Could you check a few things on this drawing? It's one solid part, dimensions in mm from its lowest x, y, z. Round coordinates to 2 decimals unless told otherwise and drop trailing zeros. Order: outer loops, then holes, each group sorted by start corner. A loop starts at its lowest first (then second) coordinate and runs counter-clockwise, first axis right, second up. Notation, with made-up numbers: (-19, 80) -> (6, 80) arc R12 cw to (6, 86) -> close; hole circle Ø1 at (33.5, 86.25). An arc over 180 degrees is marked (long way). Use a Markdown table: item, result. Add a question column.
(1) I want a section at B-B, the plane x = 2.25. Give the number of separate pieces and of enclosed holes in the cut face, then the cut area to 3 significant figures.
(2) If I drill on probe 1 along Y at (x, z) = (5, 6.5); probe 2 along Y at (x, z) = (2.75, 5); probe 3 along Z at (x, y) = (6, 15), over which ranges is the centre line in solid material (lowest first)?
(3) Thinking about a two-plate mould opening in Z: for the marked faces 1, 2, 3 and 4, which applies, pulls with the +Z half, pulls with the -Z half, needs draft (parallel to the pull), parting line crosses it, or undercut?
(4) I want a section at A-A, the plane y = 5.08. Please give me the cut outline in (x, z).
(5) I want a section at C-C, the plane y = 12.75. Please give me the cut outline in (x, z), then the cut area to 3 significant figures.
(6) I'm going to push a flat-ended pin straight in: P1, Ø3, axis at y = 5.08, z = 5.969, coming from the +X side. Where does the tip first touch, or does it pass through?
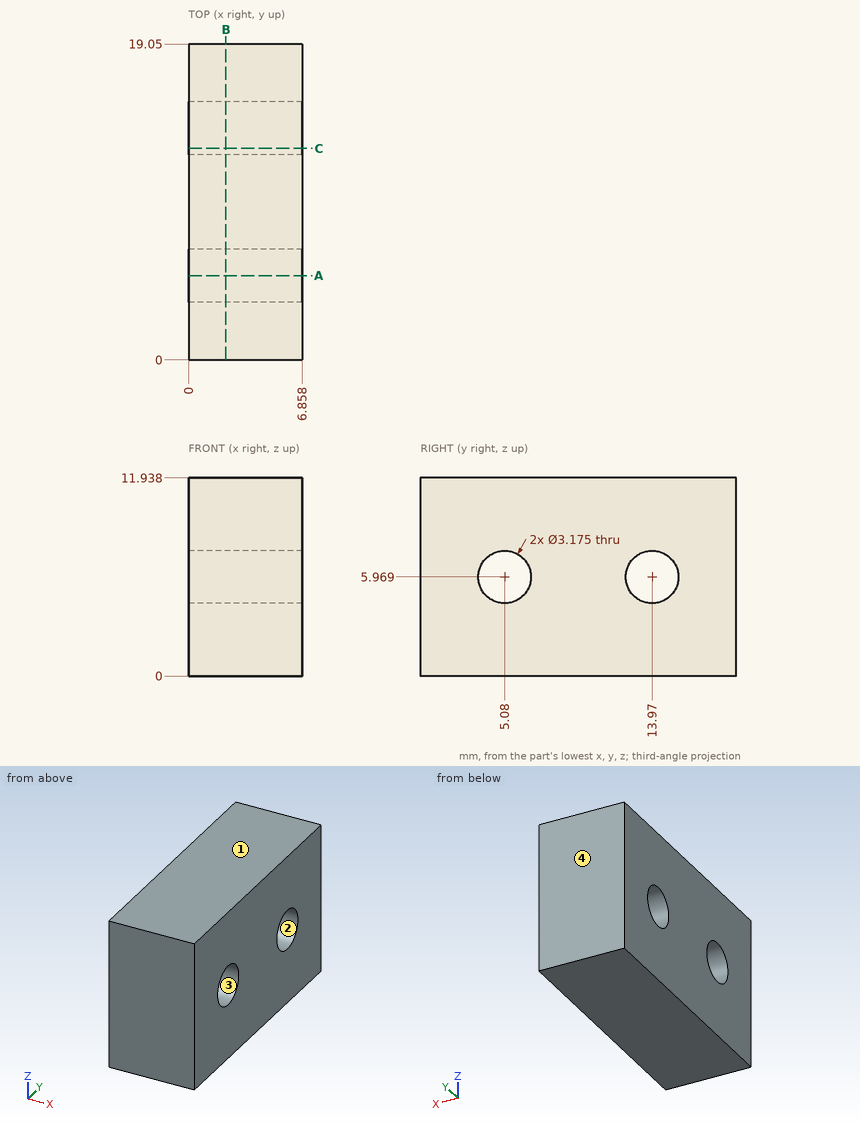
Taken from the geometry:
| question | item | result |
|---|---|---|
| 1 | separate pieces | 1 |
| 1 | enclosed holes | 2 |
| 1 | area | 212 mm2 |
| 2 | probe 1 | y = 0 to 3.58, 6.58 to 12.47, 15.47 to 19.05 |
| 2 | probe 2 | y = 0 to 3.82, 6.34 to 12.71, 15.23 to 19.05 |
| 2 | probe 3 | z = 0 to 4.76, 7.18 to 11.94 |
| 3 | face 1 | pulls with the +Z half |
| 3 | face 2 | undercut |
| 3 | face 3 | undercut |
| 3 | face 4 | needs draft |
| 4 | outline | (0, 0) -> (6.86, 0) -> (6.86, 4.38) -> (0, 4.38) -> close; (0, 7.56) -> (6.86, 7.56) -> (6.86, 11.94) -> (0, 11.94) -> close |
| 5 | outline | (0, 0) -> (6.86, 0) -> (6.86, 4.95) -> (0, 4.95) -> close; (0, 6.98) -> (6.86, 6.98) -> (6.86, 11.94) -> (0, 11.94) -> close |
| 5 | area | 67.9 mm2 |
| 6 | P1 | passes through |
